```python
from build123d import *

# Parameters (mm, degrees)
EXTRUDE_1_DEPTH     = 36
SKETCH_2_R          = 9.25
CUT_EXTRUDE_1_DEPTH = 12
SKETCH_3_R          = 1.5
CUT_EXTRUDE_2_DEPTH = 54
SKETCH_5_R          = 1.5
CUT_EXTRUDE_4_DEPTH = 10
CUT_EXTRUDE_5_DEPTH = 57
FILLET_1_R          = 5


with BuildPart() as part:
    # 草图1 → 凸台-拉伸1 (new body)
    with BuildSketch(Plane.XY):
        Polygon((0, 0), (0, 25), (2, 25), (2, 2), (33, 2), (33, 25), (35, 25), (35, 0), align=None)
    extrude(amount=EXTRUDE_1_DEPTH)

    # 草图2 → 切除-拉伸1 (cut)
    with BuildSketch(Plane.XZ):
        with Locations(Location((17.5, 18, 0), (0, 0, 270))):
            Circle(SKETCH_2_R)
    extrude(amount=-CUT_EXTRUDE_1_DEPTH, mode=Mode.SUBTRACT)

    # 草图3 → 切除-拉伸2 (cut)
    with BuildSketch(Plane.ZY):
        with Locations((18, 20.9)):
            Circle(SKETCH_3_R)
        with Locations((18, 9.7)):
            Circle(SKETCH_3_R)
    extrude(amount=-CUT_EXTRUDE_2_DEPTH, mode=Mode.SUBTRACT)

    # 草图5 → 切除-拉伸4 (cut)
    with BuildSketch(Plane(origin=(0, 2, 0), x_dir=(1, 0, 0), z_dir=(0, 1, 0))):
        with Locations(Location((8, -3.5, 0), (0, 0, 180))):
            Circle(SKETCH_5_R)
        with Locations(Location((27, -3.5, 0), (0, 0, 180))):
            Circle(SKETCH_5_R)
        with Locations(Location((8, -32.5, 0), (0, 0, 180))):
            Circle(SKETCH_5_R)
        with Locations(Location((27, -32.5, 0), (0, 0, 180))):
            Circle(SKETCH_5_R)
    extrude(amount=-CUT_EXTRUDE_4_DEPTH, mode=Mode.SUBTRACT)

    # 草图6 → 切除-拉伸5 (cut)
    with BuildSketch(Plane.ZY):
        Polygon((0, 9), (13, 25), (0, 25), align=None)
        Polygon((36, 25), (36, 9), (23, 25), align=None)
    extrude(amount=-CUT_EXTRUDE_5_DEPTH, mode=Mode.SUBTRACT)

    # 圆角1
    fillet_1_edges = [part.edges().sort_by_distance(p)[0] for p in [
        (34, 25, 13),
        (1, 25, 13),
        (34, 25, 23),
        (1, 25, 23),
    ]]
    fillet(fillet_1_edges, radius=FILLET_1_R)


solid = part.part
```
The listing builds one solid part. Answer for the finished solid, in the listing's coordinates (mm). A direction names the side the tool comes from. Give positions to 0.01 mm unless a question says otherwise; leave off trailing zeros. Order: outer loops, then holes, each group sorted by start corner. A loop starts at its lowest first (then second) coordinate and runs counter-clockwise, first axis right, second up. Notation, with made-up numbers: (9, 24.25) -> (64, 24.25) arc R15 cw to (64, 43.25) -> close; hole circle Ø6 at (-8, 39.25). An arc over 180 degrees is marked (long way). Answer as a JSON object with one key per item and string values. Group by question number.
Item 1: The part is cut by section B-B on z = 4. Write down the section's boundary in (x, y).
Item 2: A tool of negligible diameter and unlimited length cuts with its end or side. For faces 4 (the flat face through (35, 13, 18)), 5 (the flat face through (33, 13, 18)), from which of +Z, -Z, +X, -X, +Y, -Y can it reach the whole face along a straight path? Write none if from no direction.
Item 3: The part is cut by section C-C on y = 9.7. Write down the section's boundary in (x, z), and give its area (3 significant figures).
Item 4: The part is cut by section D-D on z = 32.5. Write down the section's boundary in (x, y), and give its area (3 significant figures).
Item 5: The part is cut by section A-A on x = 17.5. Write down the section's boundary in (y, z).
Item 6: Flat-ended cylindrical pins translate along their axes: pin 1 (16.5 mm diameter, centred on x = 17.5, z = 18, fed in from +Y); pin 2 (2 mm diameter, centred on x = 31, z = 8, fed in from +Y). Find the tip coordinate at first contact, or state that the pin passes through.
Item 7: Consider L1, parallel to X at y = 6, z = 18.5; L2, parallel to Z at x = 8, y = 0.8; L3, parallel to Y at x = 13.5, z = 32. Determine where each line is inside the solid, lowest interval first. Write a range as from..to.
Item 8: Determine the mould class of faces 1 (the cylindrical face through (34, 24.5, 22.8)), 2 (the cylindrical face through (33.99, 20.97, 16.5)), 3 (the flat face through (0, 12, 18)) for opening direction Z: pulls with the +Z half, pulls with the -Z half, needs draft (parallel to the pull), parting line crosses it, or undercut.
Result set:
{
 "1": {"outline": "(0, 0) -> (6.59, 0) -> (6.59, 2) -> (2, 2) -> (2, 13.92) -> (0, 13.92) -> close; (9.41, 0) -> (25.59, 0) -> (25.59, 2) -> (9.41, 2) -> close; (28.41, 0) -> (35, 0) -> (35, 13.92) -> (33, 13.92) -> (33, 2) -> (28.41, 2) -> close"},
 "2": {"face 4": "+Z, -Z, +X, +Y, -Y", "face 5": "+Z, -Z, +Y"},
 "3": {"outline": "(0, 0.57) -> (2, 0.57) -> (2, 16.5) -> (0, 16.5) -> close; (0, 19.5) -> (2, 19.5) -> (2, 35.43) -> (0, 35.43) -> close; (33, 0.57) -> (35, 0.57) -> (35, 16.5) -> (33, 16.5) -> close; (33, 19.5) -> (35, 19.5) -> (35, 35.43) -> (33, 35.43) -> close", "area": "127 mm²"},
 "4": {"outline": "(0, 0) -> (6.5, 0) -> (6.5, 2) -> (2, 2) -> (2, 13.31) -> (0, 13.31) -> close; (9.5, 0) -> (25.5, 0) -> (25.5, 2) -> (9.5, 2) -> close; (28.5, 0) -> (35, 0) -> (35, 13.31) -> (33, 13.31) -> (33, 2) -> (28.5, 2) -> close", "area": "103 mm²"},
 "5": {"outline": "(0, 0) -> (2, 0) -> (2, 8.75) -> (0, 8.75) -> close; (0, 27.25) -> (2, 27.25) -> (2, 36) -> (0, 36) -> close"},
 "6": {"pin 1": "through", "pin 2": "y = 2"},
 "7": {"L1": "0..2, 33..35", "L2": "0..2, 5..31, 34..36", "L3": "0..2"},
 "8": {"face 1": "pulls with the +Z half", "face 2": "undercut", "face 3": "needs draft"}
}
